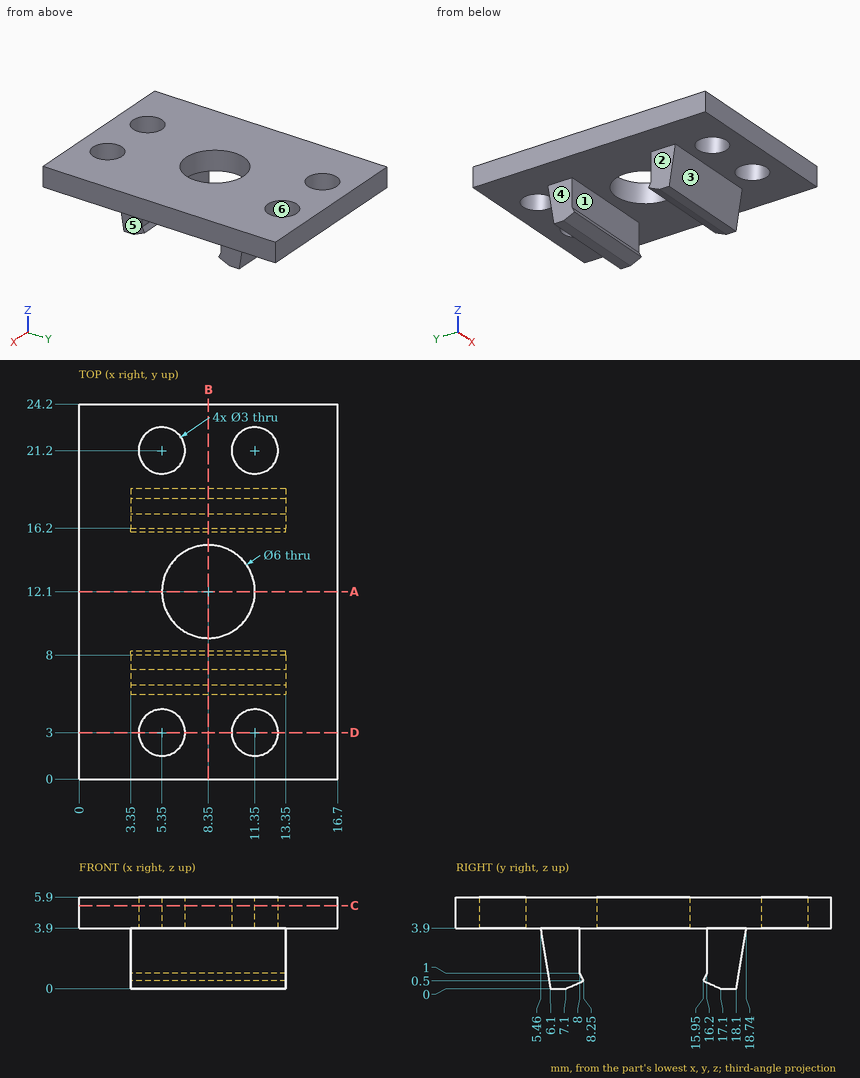
Job drawing, mm, ordinate dimensions from the low corner. One solid piece. A direction names the side the tool comes from. Give positions to 0.01 mm unless a question says otherwise; leave off trailing zeros. Order: outer loops, then holes, each group sorted by start corner. A loop starts at its lowest first (then second) coordinate and runs counter-clockwise, first axis right, second up. Notation, with made-up numbers: M -5,32 L 11,32 A30 cw 11,71 Z; hole C -32.75,-34 d11. An arc over 180 degrees is marked long. Put each result on its own line as item: value. Start each with the question number.
(1) Band-saw the part on C-C on z = 5.35. Give the cut face in (x, y).
(2) Band-saw the part on A-A on y = 12.1. Give the cut face in (x, z).
(3) Pull direction Z, two halves, no side cores. Call the marked faces 1, 2 and 3: released by +Z, released by -Z, zero draft, split by the parting line, or undercut.
(4) Tool access for the marked faces 4, 5 and 6: list every direction of +Z, -Z, +X, -X, +Y, -Y with a clear straight run to the whole face (end or side of a thin tool).
(5) Drill centre lines: L1, parallel to X at y = 12, z = 5.1; L2, parallel to Y at x = 8.35, z = 5.45; L3, parallel to X at y = 3.5, z = 5.65. Where is each one in solid material? Low to high. Write a range as [from, to].
(6) Band-saw the part on B-B on x = 8.35. Give the cut face in (y, z).
(7) Pin check, flat tips, straight feed: pin 1 Ø3.5 at (x, y) = (11.35, 3) entering from -Z; pin 2 Ø4 at (x, y) = (7.5, 14.5) entering from -Z; pin 3 Ø1.4 at (y, z) = (7.5, 2.5) entering from +X. Stop position of each tip, or through.
(8) Band-saw the part on D-D on y = 3. Give the cut face in (x, z).
Results below:
1. outline: M 0,0 L 16.7,0 L 16.7,24.2 L 0,24.2 Z; hole C 5.35,3 d3; hole C 5.35,21.2 d3; hole C 8.35,12.1 d6; hole C 11.35,3 d3; hole C 11.35,21.2 d3
2. outline: M 0,3.9 L 5.35,3.9 L 5.35,5.9 L 0,5.9 Z; M 11.35,3.9 L 16.7,3.9 L 16.7,5.9 L 11.35,5.9 Z
3. face 1: undercut
3. face 2: zero draft
3. face 3: released by -Z
4. face 4: -Z, -X, +Y, -Y
4. face 5: -Z, +X, +Y, -Y
4. face 6: +Z, -Z
5. L1: x = [0, 5.35], [11.35, 16.7]
5. L2: y = [0, 9.1], [15.1, 24.2]
5. L3: x = [0, 3.94], [6.76, 9.94], [12.76, 16.7]
6. outline: M 0,3.9 L 5.46,3.9 L 6.1,0 L 7.1,0 L 8.25,0.5 L 8,1 L 8,3.9 L 9.1,3.9 L 9.1,5.9 L 0,5.9 Z; M 15.1,3.9 L 16.2,3.9 L 16.2,1 L 15.95,0.5 L 17.1,0 L 18.1,0 L 18.74,3.9 L 24.2,3.9 L 24.2,5.9 L 15.1,5.9 Z
7. pin 1: stops at z = 3.9
7. pin 2: stops at z = 0.26
7. pin 3: stops at x = 13.35
8. outline: M 0,3.9 L 3.85,3.9 L 3.85,5.9 L 0,5.9 Z; M 6.85,3.9 L 9.85,3.9 L 9.85,5.9 L 6.85,5.9 Z; M 12.85,3.9 L 16.7,3.9 L 16.7,5.9 L 12.85,5.9 Z
